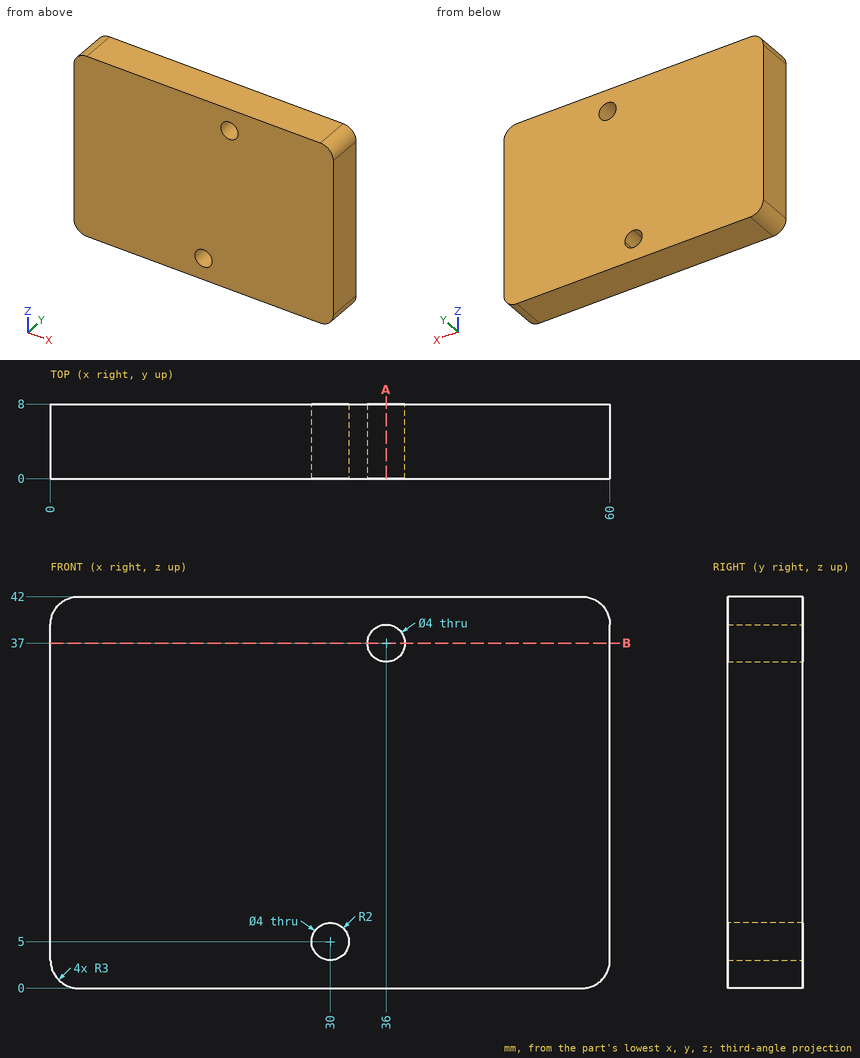
Design review of the part shown in the three views and the two pictorial views. Dimensions are in mm from the part's minimum x, y and z. Round coordinates to 2 decimals unless told otherwise and drop trailing zeros. Order: outer loops, then holes, each group sorted by start corner. A loop starts at its lowest first (then second) coordinate and runs counter-clockwise, first axis right, second up. Notation, with made-up numbers: (32.5, 24) - (65.5, 24) arc R35 cw to (65.5, 59) - close; hole circle Ø10 at (22.25, 72.25). An arc over 180 degrees is marked (long way). Answer in a Markdown table with one row per item.
(1) Take a section at A-A on x = 36. Write out the cut boundary in (y, z), plus the area to 3 significant figures.
Result set:
| item | result |
|---|---|
| outline | (0, 0) - (8, 0) - (8, 35) - (0, 35) - close; (0, 39) - (8, 39) - (8, 42) - (0, 42) - close |
| area | 304 mm2 |
(2) Clearance check with a flat-ended pin moving along its axis: P1, Ø3.5, axis at x = 36, z = 37, coming from the +Y side. State where the tip first meets the part, or that it passes through.
Result set:
| item | result |
|---|---|
| P1 | passes through |
(3) For line 1 (Z direction, x = 36, y = 7); line 2 (Z direction, x = 30, y = 2.25); line 3 (X direction, y = 2.25, z = 5), list the stretches that pass through material, from the lowest coordinate up. Write a range as from..to.
Result set:
| item | result |
|---|---|
| line 1 | z = 0..35, 39..42 |
| line 2 | z = 0..3, 7..42 |
| line 3 | x = 0..28, 32..60 |
(4) Take a section at B-B on z = 37. Write out the cut boundary in (x, y), plus the area to 3 significant figures.
Result set:
| item | result |
|---|---|
| outline | (0, 0) - (34, 0) - (34, 8) - (0, 8) - close; (38, 0) - (60, 0) - (60, 8) - (38, 8) - close |
| area | 448 mm2 |
